The drawing under review shows one solid part. Ordinate dimensions are in mm from its lowest x, y, z. A direction names the side the tool comes from. Coordinates: 2 decimals unless noted, no trailing zeros. Write each loop counter-clockwise with the first axis right and the second up, starting at its lowest first coordinate (ties: lowest second). Pieces come first, ordered by that corner, then holes. Notation, with made-up numbers: (10, 49.5) -> (28, 49.5) arc R16 cw to (28, 69.5) -> close; hole circle Ø5 at (3, 73). An arc over 180 degrees is marked (long way). Put each result on its own line as item: value. Start each with the question number.
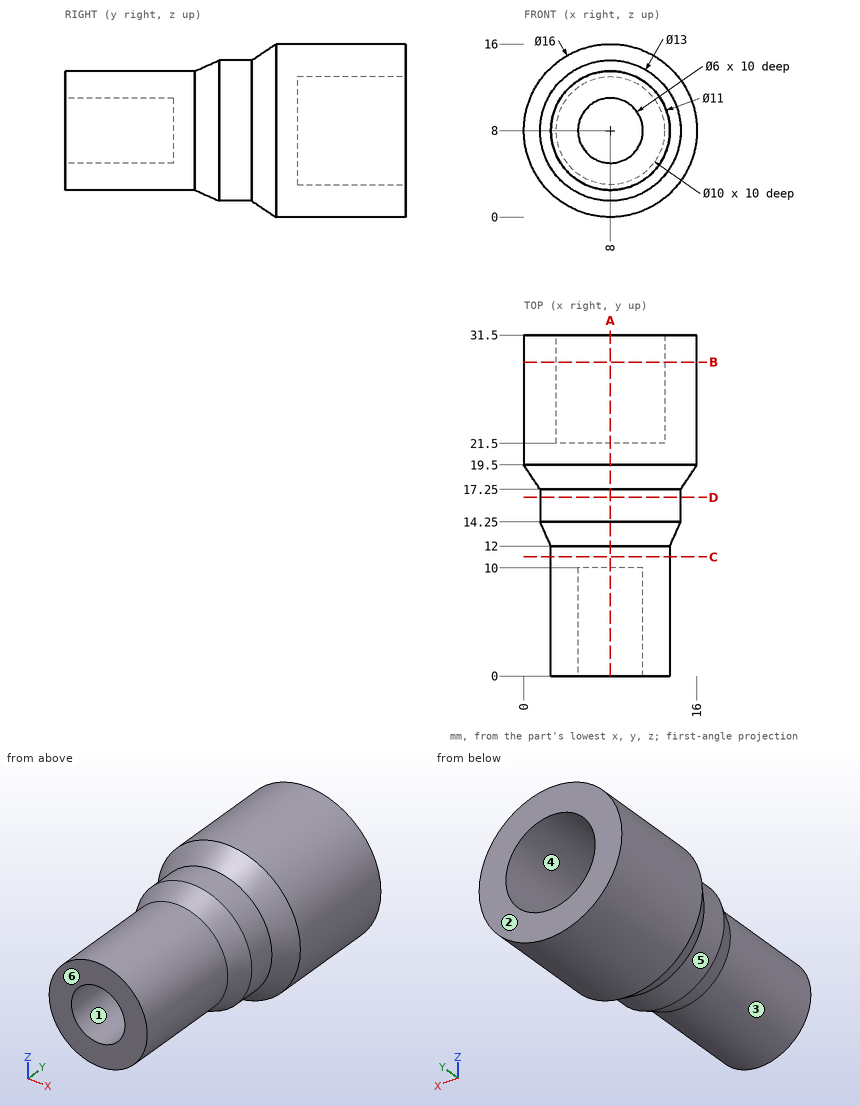
1. Wall thickness on line 1 (Z direction, x = 8, y = 25); line 2 (Z direction, x = 8, y = 6.5); line 3 (Y direction, x = 5.5, z = 9.5): over which ranges is each line inside the solid? List them lowest first. Write a range as from..to.
2. Consider section D-D on y = 16.5. State the section outline as (x, z) points.
3. Consider section B-B on y = 29. State the section outline as (x, z) points.
4. Consider section C-C on y = 11. State the section outline as (x, z) points, then the cut area to 3 significant figures.
5. Consider section A-A on x = 8. State the section outline as (y, z) points, then the cut area to 3 significant figures.
6. Insertion check: P1, Ø4, axis at x = 11.5, y = 27.5, coming from the -Z side; P2, Ø1.5, axis at x = 10, z = 6.5, coming from the +Y side; P3, Ø5.5, axis at x = 8, z = 8, coming from the -Y side. Each pin has a flat end and moves straight along its axis. Give the tip position at first contact, or say it passes through.
7. The part is to be moulded in two halves that separate along Z. For the marked faces 1, 2, 3 and 4, say which applies: released by +Z, released by -Z, zero draft, split by the parting line, or undercut.
8. Tool access review of the marked faces 5 and 6: name each direction out of +Z, -Z, +X, -X, +Y, -Y from which nothing blocks a thin tool from reaching the whole face with its end or side.
Output values:
1. line 1: z = 0..3, 13..16
1. line 2: z = 2.5..5, 11..13.5
1. line 3: y = 10..21.5
2. outline: circle Ø13 at (8, 8)
3. outline: circle Ø16 at (8, 8); hole circle Ø10 at (8, 8)
4. outline: circle Ø11 at (8, 8)
4. area: 95.0 mm^2
5. outline: (0, 2.5) -> (12, 2.5) -> (14.25, 1.5) -> (17.25, 1.5) -> (19.5, 0) -> (31.5, 0) -> (31.5, 3) -> (21.5, 3) -> (21.5, 13) -> (31.5, 13) -> (31.5, 16) -> (19.5, 16) -> (17.25, 14.5) -> (14.25, 14.5) -> (12, 13.5) -> (0, 13.5) -> (0, 11) -> (10, 11) -> (10, 5) -> (0, 5) -> close
5. area: 263 mm^2
6. P1: stops at z = 0.14
6. P2: stops at y = 21.5
6. P3: stops at y = 10
7. face 1: undercut
7. face 2: zero draft
7. face 3: split by the parting line
7. face 4: undercut
8. face 5: -Y
8. face 6: +Z, -Z, +X, -X, -Y
